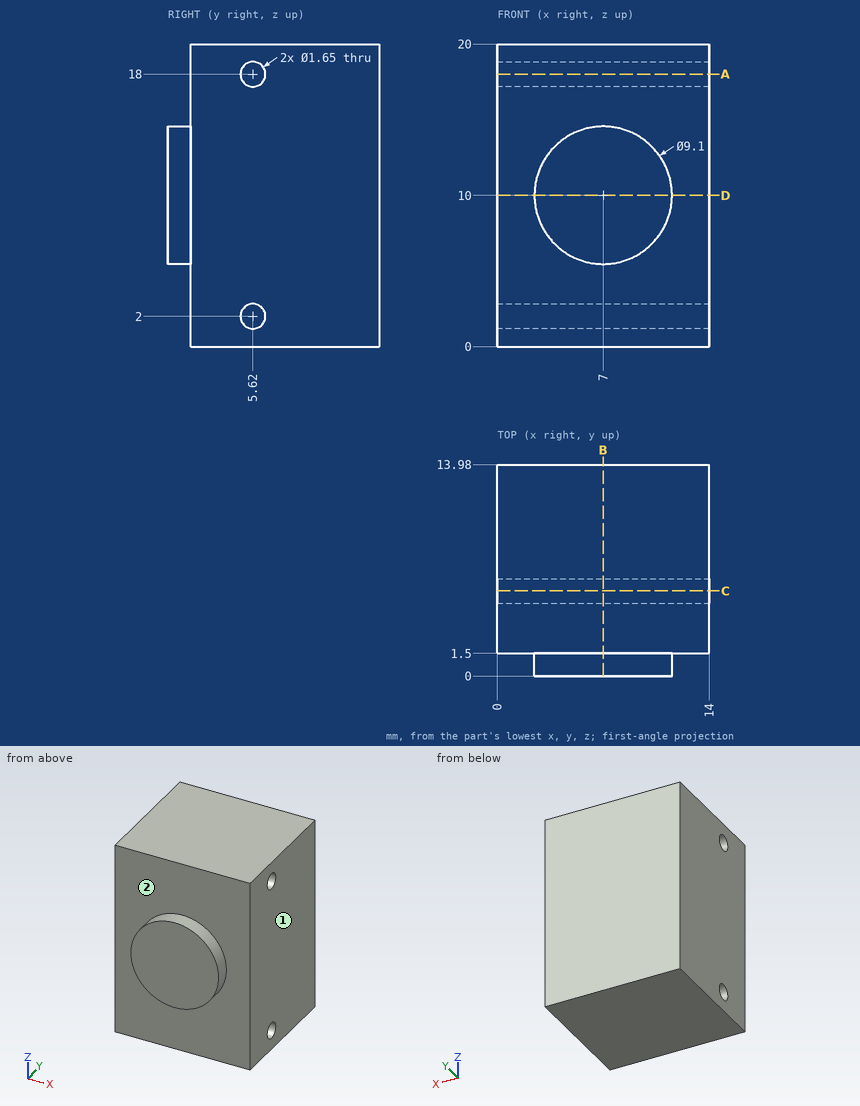
Could you check a few things on this drawing? It's one solid part, dimensions in mm from its lowest x, y, z. A direction names the side the tool comes from. Coordinates: 2 decimals unless noted, no trailing zeros. Loops run counter-clockwise (first coordinate to the right, second up) from the corner with the lowest first, then second, coordinate; pieces in that order, holes last. Notation, with made-up numbers: (-28.5, 22) - (15.5, 22) arc R12 ccw to (15.5, 43) - close; hole circle Ø1 at (-12, -30.75). An arc over 180 degrees is marked (long way). Answer as a JSON object with one key per item and string values. Group by question number.
Item 1: If we section it at B-B (x = 7): List the corners of the cut face in (y, z) for me (3 decimals), plus the area to 3 significant figures.
Item 2: On a 3-axis mill with a long thin cutter (end or side, diameter ignored), from which of +Z, -Z, +X, -X, +Y, -Y can I reach the whole of each face in a straight line? I mean the marked faces 1 and 2. Say none if no direction works.
Item 3: If we section it at A-A (z = 18): List the corners of the cut face in (x, y) for me (3 decimals), plus the area to 3 significant figures.
Item 4: If I drill on L1, parallel to Y at x = 5.25, z = 18 (3 decimals); L2, parallel to Y at x = 1.25, z = 7.75; L3, parallel to Y at x = 8, z = 18.5, over which ranges is the centre line in solid material (lowest first)? Write a range as from..to.
Item 5: For pin 1 (1 mm diameter, centred on y = 5.62, z = 2, fed in from +X), with a flat end and sliding along its axis, tell me the tip position at first contact or that it passes through.
Item 6: If we section it at D-D (z = 10): List the corners of the cut face in (x, y) for me.
Item 7: If we section it at C-C (y = 5.62): List the corners of the cut face in (x, z) for me (3 decimals).
Returned:
{
 "1": {"outline": "(0, 5.45) - (1.5, 5.45) - (1.5, 0) - (13.98, 0) - (13.98, 20) - (1.5, 20) - (1.5, 14.55) - (0, 14.55) - close; hole circle Ø1.65 at (5.62, 2); hole circle Ø1.65 at (5.62, 18)", "area": "259 mm²"},
 "2": {"face 1": "+Z, -Z, +X, +Y, -Y", "face 2": "-Y"},
 "3": {"outline": "(0, 1.5) - (14, 1.5) - (14, 4.795) - (0, 4.795) - close; (0, 6.445) - (14, 6.445) - (14, 13.98) - (0, 13.98) - close", "area": "152 mm²"},
 "4": {"L1": "y = 1.5..4.795, 6.445..13.98", "L2": "y = 1.5..13.98", "L3": "y = 1.5..4.96, 6.28..13.98"},
 "5": {"pin 1": "passes through"},
 "6": {"outline": "(0, 1.5) - (2.45, 1.5) - (2.45, 0) - (11.55, 0) - (11.55, 1.5) - (14, 1.5) - (14, 13.98) - (0, 13.98) - close"},
 "7": {"outline": "(0, 0) - (14, 0) - (14, 1.175) - (0, 1.175) - close; (0, 2.825) - (14, 2.825) - (14, 17.175) - (0, 17.175) - close; (0, 18.825) - (14, 18.825) - (14, 20) - (0, 20) - close"}
}
